from build123d import *

# Parameters (mm, degrees)
SCHIZZO1_R                   = 10.000000000000002
ESTRUSIONE_ESTRUSIONE1_DEPTH = 55
SCHIZZO2_R                   = 17.500000000000004
ESTRUSIONE_ESTRUSIONE2_DEPTH = 10
SCHIZZO3_R                   = 85.905
ESTRUSIONE_ESTRUSIONE3_DEPTH = 5
ESTRUSIONE_ESTRUSIONE4_DEPTH = 15
TAGLIO_ESTRUSIONE1_DEPTH     = 141.2117614538809
ESTRUSIONE_ESTRUSIONE5_START = 15
SCHIZZO6_R                   = 65.50000000000003
SCHIZZO6_R_2                 = 61.50000000000001
ESTRUSIONE_ESTRUSIONE5_DEPTH = 15
TAGLIO_ESTRUSIONE2_DEPTH     = 141.2117614538809
TAGLIO_ESTRUSIONE3_DEPTH     = 15
SCHIZZO9_R                   = 3.0000000000000018
TAGLIO_ESTRUSIONE4_DEPTH     = 141.2117614538809


with BuildPart() as part:
    # Schizzo1 → Estrusione-Estrusione1 (new body)
    with BuildSketch(Plane.XY):
        Circle(SCHIZZO1_R)
    extrude(amount=ESTRUSIONE_ESTRUSIONE1_DEPTH)

    # Schizzo2 → Estrusione-Estrusione2 (add)
    with BuildSketch(Plane.XY.offset(55)):
        Circle(SCHIZZO2_R)
    extrude(amount=ESTRUSIONE_ESTRUSIONE2_DEPTH)

    # Schizzo3 → Estrusione-Estrusione3 (add)
    with BuildSketch(Plane.XY.offset(65)):
        Circle(SCHIZZO3_R)
    extrude(amount=ESTRUSIONE_ESTRUSIONE3_DEPTH)

    # Schizzo4 → Estrusione-Estrusione4 (add)
    with BuildSketch(Plane.XY.offset(70)):
        with BuildLine():
            ThreePointArc((2.33238e-12, 85.905), (-40.99032330010046, 75.49478406322679), (-72.04599513935142, 46.78721630296627))
            Line((-72.0459951393514, 46.78721630296625), (-69.71449096046315, 45.27311978562447))
            ThreePointArc((-69.71449096046314, 45.27311978562449), (-39.66382194658025, 73.05167249002571), (-1.12081e-12, 83.125))
            Line((0, 83.125), (0, 85.905))
        make_face()
        with BuildLine():
            Line((10.130389170552856, -82.5053988551849), (10.469185945219174, -85.26467715674777))
            ThreePointArc((10.469185945219136, -85.26467715674778), (64.3390411943792, -56.92237524197296), (85.905, -2.104e-14))
            ThreePointArc((85.905, 0), (60.74400803783119, 60.74400803782954), (2.33238e-12, 85.905))
            Line((0, 85.905), (0, 83.125))
            ThreePointArc((-1.10236e-12, 83.125), (58.77825118613137, 58.77825118613215), (83.125, 0))
            ThreePointArc((83.125, -2.036e-14), (62.25694429058578, -55.08029150793321), (10.130389170552828, -82.5053988551849))
        make_face()
    extrude(amount=ESTRUSIONE_ESTRUSIONE4_DEPTH)

    # Schizzo5 → Taglio-Estrusione1 (cut, through all)
    with BuildSketch(Plane.XY.offset(70)):
        with BuildLine():
            Line((-69.7144909604632, 45.27311978562441), (-72.04599513935146, 46.78721630296619))
            ThreePointArc((-72.04599513935142, 46.787216302966286), (-72.85157170031785, -45.522714393953365), (10.469185945219396, -85.26467715674775))
            Line((10.469185945218987, -85.26467715674781), (10.130389170552684, -82.50539885518494))
            Line((10.130389170552684, -82.50539885518494), (7.982441993037, -65.0117729325066))
            ThreePointArc((7.9824419930370025, -65.01177293250663), (-55.54715029824602, -34.70971180727477), (-54.932922200425146, 35.67385679348449))
            Line((-54.93292220042516, 35.67385679348449), (-69.7144909604632, 45.27311978562441))
        make_face()
    extrude(amount=-TAGLIO_ESTRUSIONE1_DEPTH, mode=Mode.SUBTRACT)

    # Schizzo6 → Estrusione-Estrusione5 (add)
    with BuildSketch(Plane.XY.offset(70).offset(ESTRUSIONE_ESTRUSIONE5_START)):
        Circle(SCHIZZO6_R)
        Circle(SCHIZZO6_R_2, mode=Mode.SUBTRACT)
    extrude(amount=-ESTRUSIONE_ESTRUSIONE5_DEPTH)

    # Schizzo7 → Taglio-Estrusione2 (cut, through all)
    with BuildSketch(Plane.XY.offset(70)):
        with BuildLine():
            Line((-9.094792559402517, 55.53858792138523), (-3.5451694376210634, 21.649059417410207))
            ThreePointArc((-3.5451694376210634, 21.649059417410207), (-4.118256573097941, 18.39563458554113), (-6.595126237509526, 16.209698020361557))
            ThreePointArc((-6.595126237509526, 16.209698020361557), (-7.944833745441985, 15.59261417329648), (-9.237403232743027, 14.863390646676436))
            ThreePointArc((-9.237403232743027, 14.863390646676436), (-12.461730523190647, 14.144422270775147), (-15.430658668606016, 15.59310017453149))
            Line((-15.430658668606016, 15.59310017453149), (-39.58587653291128, 40.00260465421101))
            ThreePointArc((-39.58587653291128, 40.00260465421101), (-41.025744459915046, 43.76718552220088), (-39.2205410364265, 47.37086827164967))
            ThreePointArc((-39.2205410364265, 47.37086827164967), (-27.92041573398183, 54.796901237584784), (-15.27058186191767, 59.57398198541434))
            ThreePointArc((-15.27058186191767, 59.57398198541434), (-11.294069325563324, 58.91623065925357), (-9.094792559402517, 55.53858792138523))
        make_face()
        with BuildLine():
            Line((43.550431750534024, 35.64561535928479), (16.976050704705482, 13.894736502405099))
            ThreePointArc((16.976050704705482, 13.894736502405099), (13.871958583265304, 12.764332104375594), (10.740447154552704, 13.816395873029286))
            ThreePointArc((10.740447154552704, 13.816395873029286), (9.53118311276309, 14.676734939044845), (8.253372270022329, 15.431521187894159))
            ThreePointArc((8.253372270022329, 15.431521187894159), (6.018563746750371, 17.864386343586606), (5.788691540596875, 21.159892491405103))
            Line((5.788691540596875, 21.159892491405103), (14.850333581636846, 54.28367703568089))
            ThreePointArc((14.850333581636846, 54.28367703568089), (17.390622284415066, 57.41292967255552), (21.41410480436174, 57.65141902354019))
            ThreePointArc((21.41410480436174, 57.65141902354019), (33.495300653424565, 51.578239928643306), (43.95729087300659, 43.011702815697646))
            ThreePointArc((43.95729087300659, 43.011702815697646), (45.37591778335563, 39.239066277667106), (43.550431750534024, 35.64561535928479))
        make_face()
        with BuildLine():
            Line((52.645224309936374, -19.89297256210059), (20.52122014232648, -7.754322915005166))
            ThreePointArc((20.52122014232648, -7.754322915005166), (17.990215156363192, -5.631302481165585), (17.335573392062187, -2.3933021473323244))
            ThreePointArc((17.335573392062187, -2.3933021473323244), (17.476016858205035, -0.9158792342516949), (17.49077550276533, 0.5681305412176627))
            ThreePointArc((17.49077550276533, 0.5681305412176627), (18.480294269940998, 3.7199640728113863), (21.21935020920287, 5.566792316873533))
            Line((21.21935020920287, 5.566792316873533), (54.436210114548075, 14.281072381469665))
            ThreePointArc((54.436210114548075, 14.281072381469665), (58.416366744330055, 13.64574415035441), (60.634645840788174, 10.280550751890294))
            ThreePointArc((60.634645840788174, 10.280550751890294), (61.41571638740626, -3.2186613089416714), (59.2278727349241, -16.562279169716877))
            ThreePointArc((59.2278727349241, -16.562279169716877), (56.66998710891878, -19.67716438158663), (52.645224309936374, -19.89297256210059))
        make_face()
        with BuildLine():
            Line((9.094792559402126, -55.538587921385286), (3.54516943762091, -21.649059417410225))
            ThreePointArc((3.54516943762091, -21.649059417410225), (4.118256573097811, -18.395634585541153), (6.595126237509411, -16.209698020361596))
            ThreePointArc((6.595126237509411, -16.209698020361596), (7.944833745441873, -15.592614173296528), (9.237403232742922, -14.863390646676493))
            ThreePointArc((9.237403232742922, -14.863390646676493), (12.461730523190546, -14.144422270775227), (15.430658668605904, -15.593100174531589))
            Line((15.430658668605904, -15.593100174531589), (39.585876532911, -40.00260465421129))
            ThreePointArc((39.585876532911, -40.00260465421129), (41.02574445991474, -43.76718552220117), (39.22054103642617, -47.37086827164993))
            ThreePointArc((39.22054103642617, -47.37086827164993), (27.92041573398144, -54.79690123758496), (15.27058186191725, -59.57398198541444))
            ThreePointArc((15.27058186191725, -59.57398198541444), (11.29406932556291, -58.91623065925364), (9.094792559402126, -55.538587921385286))
        make_face()
        with BuildLine():
            Line((-43.55043175053426, -35.645615359284484), (-16.976050704705578, -13.89473650240498))
            ThreePointArc((-16.976050704705578, -13.89473650240498), (-13.87195858326539, -12.764332104375498), (-10.740447154552799, -13.816395873029213))
            ThreePointArc((-10.740447154552799, -13.816395873029213), (-9.53118311276319, -14.676734939044781), (-8.253372270022437, -15.4315211878941))
            ThreePointArc((-8.253372270022437, -15.4315211878941), (-6.018563746750495, -17.86438634358656), (-5.7886915405970205, -21.159892491405063))
            Line((-5.7886915405970205, -21.159892491405063), (-14.850333581637225, -54.283677035680796))
            ThreePointArc((-14.850333581637225, -54.283677035680796), (-17.39062228441547, -57.41292967255541), (-21.414104804362143, -57.65141902354005))
            ThreePointArc((-21.414104804362143, -57.65141902354005), (-33.49530065342495, -51.57823992864311), (-43.9572908730069, -43.01170281569734))
            ThreePointArc((-43.9572908730069, -43.01170281569734), (-45.375917783355895, -39.23906627766678), (-43.55043175053426, -35.645615359284484))
        make_face()
        with BuildLine():
            Line((-52.64522430993622, 19.892972562100955), (-20.52122014232642, 7.754322915005307))
            ThreePointArc((-20.52122014232642, 7.754322915005307), (-17.990215156363146, 5.631302481165709), (-17.335573392062166, 2.393302147332444))
            ThreePointArc((-17.335573392062166, 2.393302147332444), (-17.47601685820502, 0.915879234251819), (-17.49077550276533, -0.5681305412175421))
            ThreePointArc((-17.49077550276533, -0.5681305412175421), (-18.480294269941023, -3.7199640728112584), (-21.219350209202908, -5.566792316873385))
            Line((-21.219350209202908, -5.566792316873385), (-54.43621011454816, -14.281072381469283))
            ThreePointArc((-54.43621011454816, -14.281072381469283), (-58.41636674433013, -13.645744150354004), (-60.63464584078823, -10.280550751889873))
            ThreePointArc((-60.63464584078823, -10.280550751889873), (-61.41571638740626, 3.218661308942107), (-59.22787273492397, 16.562279169717286))
            ThreePointArc((-59.22787273492397, 16.562279169717286), (-56.66998710891863, 19.677164381587026), (-52.64522430993622, 19.892972562100955))
        make_face()
    extrude(amount=-TAGLIO_ESTRUSIONE2_DEPTH, mode=Mode.SUBTRACT)

    # Schizzo8 → Taglio-Estrusione3 (cut)
    with BuildSketch(Plane.XY.offset(85)):
        with BuildLine():
            Line((-65.41023452642462, 3.4280051339130924), (-61.41571638740627, 3.2186613089413))
            ThreePointArc((-61.41571638740627, 3.2186613089413), (-52.15495791361932, -32.590034750342085), (-24.029964402089327, -56.61104848732551))
            Line((-24.029964402089327, -56.61104848732551), (-25.592888916046377, -60.29306790113534))
            ThreePointArc((-25.592888916046377, -60.29306790113534), (-55.547150298245406, -34.709711807275156), (-65.41023452642462, 3.4280051339130924))
        make_face()
    extrude(amount=-TAGLIO_ESTRUSIONE3_DEPTH, mode=Mode.SUBTRACT)

    # Schizzo9 → Taglio-Estrusione4 (cut, through all)
    with BuildSketch(Plane.XY.offset(70)):
        with Locations((-48.11604392732846, -24.512166709277214)):
            Circle(SCHIZZO9_R)
    extrude(amount=-TAGLIO_ESTRUSIONE4_DEPTH, mode=Mode.SUBTRACT)


solid = part.part
For this review, take the finished solid that the model builds, in its own axes (mm). A direction names the side the tool comes from. Coordinates: 2 decimals unless noted, no trailing zeros. Loops run counter-clockwise (first coordinate to the right, second up) from the corner with the lowest first, then second, coordinate; pieces in that order, holes last. Notation, with made-up numbers: (-15, 46) - (5, 46) arc R29 ccw to (5, 70) - close; hole circle Ø4 at (-27.5, 32). An arc over 180 degrees is marked (long way). Use a Markdown table: item, result. Add a question column.
Item 1: We need section A-A (x = 0). Give the boundary of the cut face in (y, z) (3 decimals), and give its area (3 significant figures).
Item 2: We need section D-D (z = 42.5). Give the boundary of the cut face in (x, y).
Item 3: Tool access review of faces 1 (the face through (-63.441, 3.325, 77.605)), 2 (the face through (8, -8, 55)), 3 (the face through (-6.36, 38.83, 67.54)), 4 (the face through (52, 44, 70)), 5 (the face through (-65.43, 42.49, 69.77)): name each direction out of +Z, -Z, +X, -X, +Y, -Y from which nothing blocks a thin tool from reaching the whole face with its end or side.
Item 4: For line 1 (Y direction, x = 0, z = 75) (3 decimals); line 2 (X direction, y = 10, z = 74); line 3 (X direction, y = 0, z = 80.25) (3 decimals), list the stretches that pass through material, from the lowest coordinate up.
Item 5: Mouldability with a two-part tool opening along Y and no side actions: class faces 6 (the face through (9.404, -76.591, 69.768)), 7 (the face through (-45.38, -39.3, 67.54)), 8 (the face through (43.4, 44, 85)), 9 (the face through (-27.34, 27.63, 67.54)) as pulls with the +Y half, pulls with the -Y half, needs draft (parallel to the pull), parting line crosses it, or undercut.
Item 6: We need section C-C (x = 32). Give the boundary of the cut face in (y, z).
Item 7: Insertion check: pin 1 Ø5 at (y, z) = (-20, 74.5) entering from -X; pin 2 Ø4 at (x, z) = (-2.5, 13.5) entering from +Y; pin 3 Ø2 at (x, y) = (-33, -27) entering from +Z; pin 4 Ø17.5 at (x, y) = (6.5, 2.5) entering from -Z. Each pin has a flat end and moves straight along its axis. Give the tip position at first contact, or say it passes through.
Results list:
| question | item | result |
|---|---|---|
| 1 | outline | (-65.5, 65) - (-17.5, 65) - (-17.5, 55) - (-10, 55) - (-10, 0) - (10, 0) - (10, 55) - (17.5, 55) - (17.5, 65) - (85.905, 65) - (85.905, 85) - (83.125, 85) - (83.125, 70) - (65.5, 70) - (65.5, 85) - (61.5, 85) - (61.5, 70) - (-61.5, 70) - (-61.5, 85) - (-65.5, 85) - close |
| 1 | area | 2,370 mm^2 |
| 2 | outline | circle Ø20 at (0, 0) |
| 3 | face 1 | +Z, -X, -Y |
| 3 | face 2 | -Z |
| 3 | face 3 | +Z, -Z |
| 3 | face 4 | +Z |
| 3 | face 5 | +Z, -Z, -X |
| 4 | line 1 | y = -65.5 to -61.5, 61.5 to 65.5, 83.125 to 85.905 |
| 4 | line 2 | x = -64.73 to -60.68, 60.68 to 64.73, 82.52 to 85.32 |
| 4 | line 3 | x = 61.5 to 65.5, 83.125 to 85.905 |
| 5 | face 6 | pulls with the -Y half |
| 5 | face 7 | undercut |
| 5 | face 8 | needs draft |
| 5 | face 9 | undercut |
| 6 | outline | (-79.72, 65) - (-52.52, 65) - (-52.52, 85) - (-57.15, 85) - (-57.15, 70) - (-76.72, 70) - (-76.72, 85) - (-79.72, 85) - close; (-32.34, 65) - (-12.09, 65) - (-12.09, 70) - (-32.34, 70) - close; (8.4, 65) - (26.19, 65) - (26.19, 70) - (8.4, 70) - close; (52.52, 65) - (79.72, 65) - (79.72, 85) - (76.72, 85) - (76.72, 70) - (57.15, 70) - (57.15, 85) - (52.52, 85) - close |
| 7 | pin 1 | stops at x = 57.24 |
| 7 | pin 2 | stops at y = 9.99 |
| 7 | pin 3 | stops at z = 70 |
| 7 | pin 4 | stops at z = 0 |
